```python
from build123d import *

# Parameters (mm, degrees)
SKETCH_2_R          = 1.6
SKETCH_2_R_2        = 17
SKETCH_2_R_3        = 1.65
EXTRUDE_2_DEPTH     = 3.5
EXTRUDE_3_DEPTH     = 18
EXTRUDE_4_DEPTH     = 10
CUT_EXTRUDE_5_DEPTH = 117.156532317
SKETCH_10_R         = 2.75
SKETCH_10_R_2       = 1.6
CUT_EXTRUDE_4_DEPTH = 5
EXTRUDE_5_DEPTH     = 18
SKETCH_14_R         = 1.55
CUT_EXTRUDE_6_DEPTH = 10


with BuildPart() as part:
    # 草图2 → 凸台-拉伸2 (new body)
    with BuildSketch(Plane(origin=(0, 0, 0), x_dir=(1, 0, 0), z_dir=(0, 1, 0))):
        Polygon((-42.5, 33.8), (-42.5, 62.8), (-27.5, 62.8), (-27.5, 53.8), (10, 53.8), (10, 62.8), (40, 62.8), (40, 53.8), (77.5, 53.8), (77.5, 62.8), (92.5, 62.8), (92.5, 33.8), (50, 33.8), (50, 0), (0, 0), (0, 33.8), align=None)
        with Locations(Location((-35, 55.312210178, 0), (0, 0, 270))):
            Circle(SKETCH_2_R, mode=Mode.SUBTRACT)
        with Locations(Location((85, 55.312210178, 0), (0, 0, 270))):
            Circle(SKETCH_2_R, mode=Mode.SUBTRACT)
        with Locations(Location((18, 55.312210178, 0), (0, 0, 270))):
            Circle(SKETCH_2_R, mode=Mode.SUBTRACT)
        with Locations(Location((32, 55.312210178, 0), (0, 0, 270))):
            Circle(SKETCH_2_R, mode=Mode.SUBTRACT)
        with Locations(Location((25, 28.8, 0), (0, 0, 270))):
            Circle(SKETCH_2_R_2, mode=Mode.SUBTRACT)
        with Locations(Location((40.5, 44.3, 0), (0, 0, 270))):
            Circle(SKETCH_2_R_3, mode=Mode.SUBTRACT)
        with Locations(Location((40.5, 13.3, 0), (0, 0, 270))):
            Circle(SKETCH_2_R_3, mode=Mode.SUBTRACT)
        with Locations(Location((9.5, 13.3, 0), (0, 0, 270))):
            Circle(SKETCH_2_R_3, mode=Mode.SUBTRACT)
        with Locations(Location((9.5, 44.3, 0), (0, 0, 270))):
            Circle(SKETCH_2_R_3, mode=Mode.SUBTRACT)
    extrude(amount=EXTRUDE_2_DEPTH)

    # 草图6 → 凸台-拉伸3 (add)
    with BuildSketch(Plane(origin=(0, 3.5, 0), x_dir=(1, 0, 0), z_dir=(0, 1, 0))):
        Polygon((10, 53.8), (-27.5, 53.8), (-27.5, 62.8), (-42.5, 62.8), (-42.5, 33.8), (0, 33.8), (0, 0), (50, 0), (50, 33.8), (92.5, 33.8), (92.5, 62.8), (77.5, 62.8), (77.5, 53.8), (40, 53.8), (40, 62.8), (10, 62.8), align=None)
        Polygon((12, 51.8), (-29.5, 51.8), (-29.5, 60.8), (-40.5, 60.8), (-40.5, 35.8), (2.5, 35.8), (2.5, 4), (47.5, 4), (47.5, 35.8), (90.5, 35.8), (90.5, 60.8), (79.5, 60.8), (79.5, 51.8), (38, 51.8), (38, 60.8), (12, 60.8), align=None, mode=Mode.SUBTRACT)
    extrude(amount=EXTRUDE_3_DEPTH)

    # 草图11 → 凸台-拉伸4 (add)
    with BuildSketch(Plane(origin=(0, 21.5, 0), x_dir=(1, 0, 0), z_dir=(0, 1, 0))):
        Polygon((2.5, 35.8), (2.5, 4), (47.5, 4), (47.5, 35.8), (50, 35.8), (50, 0), (0, 0), (0, 35.8), align=None)
    extrude(amount=EXTRUDE_4_DEPTH)

    # 草图12 → 切除-拉伸5 (cut, through all)
    with BuildSketch(Plane.ZY):
        Polygon((-35.8, 21.5), (-4, 31.5), (-35.8, 31.5), align=None)
    extrude(amount=-CUT_EXTRUDE_5_DEPTH, mode=Mode.SUBTRACT)

    # 草图10 → 切除-拉伸4 (cut)
    with BuildSketch(Plane.XY):
        with Locations((25, 15.656854249)):
            Circle(SKETCH_10_R)
        with Locations((30.656854249, 21.313708499)):
            Circle(SKETCH_10_R_2)
        with Locations((30.656854249, 10)):
            Circle(SKETCH_10_R_2)
        with Locations((19.343145751, 10)):
            Circle(SKETCH_10_R_2)
        with Locations((19.343145751, 21.313708499)):
            Circle(SKETCH_10_R_2)
    extrude(amount=-CUT_EXTRUDE_4_DEPTH, mode=Mode.SUBTRACT)

    # 草图13 → 凸台-拉伸5 (add)
    with BuildSketch(Plane(origin=(0, 3.5, 0), x_dir=(1, 0, 0), z_dir=(0, 1, 0))):
        Polygon((-12.5, 35.8), (-21.737604307, 51.8), (-24.047005384, 51.8), (-14.809401077, 35.8), align=None)
        Polygon((-3.262395693, 51.8), (-12.5, 35.8), (-10.190598923, 35.8), (-0.952994616, 51.8), align=None)
        Polygon((50.952994616, 51.8), (60.190598923, 35.8), (62.5, 35.8), (53.262395693, 51.8), align=None)
        Polygon((71.737604307, 51.8), (62.5, 35.8), (64.809401077, 35.8), (74.047005384, 51.8), align=None)
    extrude(amount=EXTRUDE_5_DEPTH)

    # 草图14 → 切除-拉伸6 (cut)
    with BuildSketch(Plane(origin=(0, 0, -62.8), x_dir=(-1, 0, 0), z_dir=(0, 0, -1))):
        with Locations((35, 15.656854249)):
            Circle(SKETCH_14_R)
        with Locations(Location((-85, 15.656854249, 0), (0, 0, 180))):
            Circle(SKETCH_14_R)
        with Locations((-25, 15.656854249)):
            Circle(SKETCH_14_R)
    extrude(amount=-CUT_EXTRUDE_6_DEPTH, mode=Mode.SUBTRACT)


solid = part.part
```
Source: CAD feature listing. Evaluate the final solid. Frame: model axes, mm. A direction names the side the tool comes from. Give positions to 0.01 mm unless a question says otherwise; leave off trailing zeros. Write each loop counter-clockwise with the first axis right and the second up, starting at its lowest first coordinate (ties: lowest second). Pieces come first, ordered by that corner, then holes. Notation, with made-up numbers: (-7, 31) - (42, 31) arc R15 ccw to (42, 48) - close; hole circle Ø8 at (7, 41.5). An arc over 180 degrees is marked (long way). One line per item, written item: value. Start each with the question number.
Q1. Material intervals for probe 1 along X at (y, z) = (17.5, -54); probe 2 along X at (y, z) = (19, -47); probe 3 along X at (y, z) = (10, -17), sorted ascending. Write a range as from..to.
Q2. Section query B-B, the plane y = 10. Count the separate pieces of the cut face and the enclosed holes in it, then the cut area to 3 significant figures.
Q3. Section query C-C, the plane x = 85. Return the cut outline in (y, z).
Q4. Draft query along X for faces 6 (the face through (-7.817, 12.374, -43.912)), 7 (the face through (25, 19, 0)), 8 (the face through (-42.5, 11, -49)), 9 (the face through (77, 12, -51.8)). Return one class per face: +X half, -X half, draft (parallel to the pull), parting line (faces both ways), or undercut.
Q5. Section query D-D, the plane z = -13.3. Return the cut outline in (x, y).
Q6. First-contact query: pin 1 Ø5 at (x, y) = (68.5, 21) entering from +Z; pin 2 Ø2 at (x, y) = (3.5, 15) entering from +Z; pin 3 Ø2.5 at (x, z) = (9.5, -44.3) entering from -Y; pin 4 Ø12 at (y, z) = (22.5, -14) entering from -X. Flat tips, straight axial feed; report the tip coordinate or a pass-through.
Q7. Set-up query: faces 1 (the face through (19.586, 1.726, -55.52)), 2 (the face through (-35, 11, -62.8)), 3 (the face through (-28, 12, -35.8)), 4 (the face through (-27.5, 11, -58)), 5 (the face through (29.06, 10.07, -1.97)). Return all of +Z, -Z, +X, -X, +Y, -Y with unobstructed straight access to the full face (end or side cutting, diameter ignored); none if empty.
Q8. Section query A-A, the plane x = 25. Return the cut outline in (y, z).
Answer:
1. probe 1: x = -42.5..-40.5, -29.5..-27.5, 10..12, 38..40, 77.5..79.5, 90.5..92.5
1. probe 2: x = -42.5..-40.5, -21.28..-18.97, -6.03..-3.72, 53.72..56.03, 68.97..71.28, 90.5..92.5
1. probe 3: x = 0..2.5, 47.5..50
2. separate pieces: 2
2. enclosed holes: 4
2. area: 1,090 mm2
3. outline: (0, -62.8) - (14.11, -62.8) - (14.11, -60.8) - (3.5, -60.8) - (3.5, -56.91) - (0, -56.91) - close; (0, -53.71) - (3.5, -53.71) - (3.5, -35.8) - (21.5, -35.8) - (21.5, -33.8) - (0, -33.8) - close; (17.21, -62.8) - (21.5, -62.8) - (21.5, -60.8) - (17.21, -60.8) - close
4. face 6: undercut
4. face 7: draft
4. face 8: -X half
4. face 9: undercut
5. outline: (0, 0) - (7.85, 0) - (7.85, 3.5) - (2.5, 3.5) - (2.5, 28.58) - (0, 28.58) - close; (11.15, 0) - (18.02, 0) - (18.02, 3.5) - (11.15, 3.5) - close; (31.98, 0) - (38.85, 0) - (38.85, 3.5) - (31.98, 3.5) - close; (42.15, 0) - (50, 0) - (50, 28.58) - (47.5, 28.58) - (47.5, 3.5) - (42.15, 3.5) - close
6. pin 1: stops at z = -33.8
6. pin 2: stops at z = 0
6. pin 3: passes through
6. pin 4: stops at x = 0
7. face 1: +Y, -Y
7. face 2: -Z, +X, -X, +Y, -Y
7. face 3: +Y
7. face 4: -Z, +Y, -Y
7. face 5: +Z
8. outline: (0, -62.8) - (14.11, -62.8) - (14.11, -60.8) - (3.5, -60.8) - (3.5, -45.8) - (0, -45.8) - close; (0, -11.8) - (3.5, -11.8) - (3.5, -4) - (12.91, -4) - (12.91, 0) - (0, 0) - close; (17.21, -62.8) - (21.5, -62.8) - (21.5, -60.8) - (17.21, -60.8) - close; (18.41, -4) - (31.5, -4) - (31.5, 0) - (18.41, 0) - close
